Geometry: final body of the model. Coordinates: model frame, mm. Face numbers are marked on the shaded views. A direction names the side the tool comes from. Give positions to 0.01 mm unless a question says otherwise; leave off trailing zeros. Write each loop counter-clockwise with the first axis right and the second up, starting at its lowest first coordinate (ties: lowest second). Pieces come first, ordered by that corner, then holes.
```python
from build123d import *

# Parameters (mm, degrees)
SKETCH1_W      = 12.7
SKETCH1_H      = 18.54
EXTRUDE1_DEPTH = 20.14
SKETCH2_W      = 15
SKETCH2_H      = 20.83
EXTRUDE2_DEPTH = 2.03
FILLET1_R      = 0.5
EXTRUDE3_DEPTH = 12.7


with BuildPart() as part:
    # Sketch1 → Extrude1 (new body)
    with BuildSketch(Plane.XY):
        with Locations((6.35, -9.27)):
            Rectangle(SKETCH1_W, SKETCH1_H)
    extrude(amount=EXTRUDE1_DEPTH)

    # Sketch2 → Extrude2 (add)
    with BuildSketch(Plane(origin=(0, 0, 0), x_dir=(-1, 0, 0), z_dir=(0, 0, -1))):
        with Locations((-6.35, -9.2725)):
            Rectangle(SKETCH2_W, SKETCH2_H)
    extrude(amount=EXTRUDE2_DEPTH)

    # Fillet1
    fillet1_edges = [part.edges().sort_by_distance(p)[0] for p in [
        (6.35, 1.1425, -2.03),
        (13.85, -9.2725, -2.03),
        (-1.15, -9.2725, -2.03),
        (6.35, -19.6875, -2.03),
    ]]
    fillet(fillet1_edges, radius=FILLET1_R)

    # Sketch3 → Extrude3 (add)
    with BuildSketch(Plane.ZY):
        with BuildLine():
            Line((-2.03, -18.257976245), (-2.03, -0.473719642))
            Line((-2.03, -0.473719642), (-5.186140292, -4.258209447))
            ThreePointArc((-5.186140292, -4.258209447), (-2.828813648, -11.082415432), (-2.03, -18.257976245))
        make_face()
    extrude(amount=-EXTRUDE3_DEPTH)


solid = part.part
```
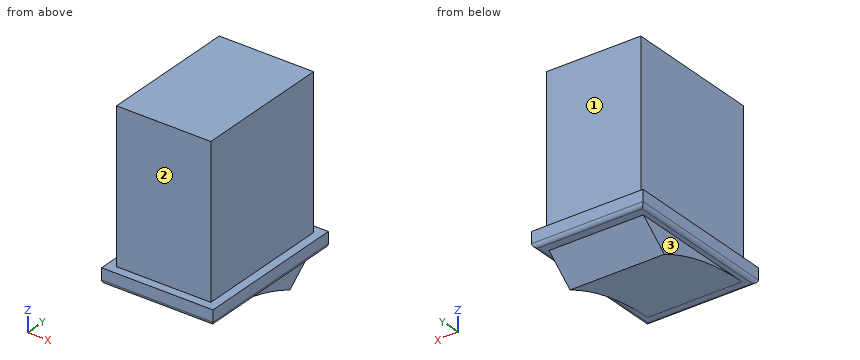
Item 1: Section C-C, the plane z = 16.5. Return the cut outline in (x, y).
Found:
outline: (0, -18.54) - (12.7, -18.54) - (12.7, 0) - (0, 0) - close
Item 2: Pin query (flat end, axial travel): pin 1 Ø3.5 at (y, z) = (-12.5, -4) entering from +X; pin 2 Ø4 at (y, z) = (-2.5, 11) entering from -X; pin 3 Ø2 at (x, z) = (9, 5) entering from +Y. Return the tip coordinate at first contact, or that it passes through.
Found:
pin 1: stops at x = 12.7
pin 2: stops at x = 0
pin 3: stops at y = 0
Item 3: Reachability of the marked faces 1, 2 and 3 from +Z, -Z, +X, -X, +Y, -Y: full face, straight path, thin tool, end or side. Return the list, or none.
Found:
face 1: +Z, +X, -X, +Y
face 2: +Z, +X, -X, -Y
face 3: -Z, -X, +Y, -Y
Item 4: Section D-D, the plane y = -11.75. Return the cut outline in (x, z).
Found:
outline: (-1.15, -1.53) arc R0.5 ccw to (-0.65, -2.03) - (0, -2.03) - (0, -2.69) - (12.7, -2.69) - (12.7, -2.03) - (13.35, -2.03) arc R0.5 ccw to (13.85, -1.53) - (13.85, 0) - (12.7, 0) - (12.7, 20.14) - (0, 20.14) - (0, 0) - (-1.15, 0) - close
Item 5: Section A-A, the plane x = 12. Return the cut outline in (y, z), plus the area to 3 significant figures.
Found:
outline: (-19.69, -1.53) arc R0.5 ccw to (-19.19, -2.03) - (-18.26, -2.03) arc R32.63 cw to (-4.26, -5.19) - (-0.47, -2.03) - (0.64, -2.03) arc R0.5 ccw to (1.14, -1.53) - (1.14, 0) - (0, 0) - (0, 20.14) - (-18.54, 20.14) - (-18.54, 0) - (-19.69, 0) - close
area: 436 mm2
Item 6: Section B-B, the plane y = -1.25. Return the cut outline in (x, z).
Found:
outline: (-1.15, -1.53) arc R0.5 ccw to (-0.65, -2.03) - (0, -2.03) - (0, -2.68) - (12.7, -2.68) - (12.7, -2.03) - (13.35, -2.03) arc R0.5 ccw to (13.85, -1.53) - (13.85, 0) - (12.7, 0) - (12.7, 20.14) - (0, 20.14) - (0, 0) - (-1.15, 0) - close
Item 7: Line query: L1, parallel to Y at x = 11, z = 9.75; L2, parallel to X at y = -13.5, z = 9.5; L3, parallel to Z at x = 13, y = -7.5. Output: solid intervals per line, ascending.
Found:
L1: y = -18.54 to 0
L2: x = 0 to 12.7
L3: z = -2.03 to 0
